Source: CAD feature listing. Evaluate the final solid. Frame: model axes, mm. Face numbers are marked on the shaded views. A direction names the side the tool comes from. Round coordinates to 2 decimals unless told otherwise and drop trailing zeros. Order: outer loops, then holes, each group sorted by start corner. A loop starts at its lowest first (then second) coordinate and runs counter-clockwise, first axis right, second up. Notation, with made-up numbers: (89.5, 15) -> (127.5, 15) arc R16 ccw to (127.5, 24) -> close; hole circle Ø5 at (23, 9). An arc over 180 degrees is marked (long way). Write item = value, one per line. Start each with the question number.
(1) Reachability of the marked faces 1, 2, 3 and 4 from +Z, -Z, +X, -X, +Y, -Y: full face, straight path, thin tool, end or side. Return the list, or none.
(2) Cut plane B-B on x = -3.5. Return the cut outline in (y, z) (3 decimals).
(3) Contact query for flat-ended pins moving along their axis: pin 1 Ø3 at (x, y) = (-2.5, 3) entering from +Z; pin 2 Ø0.7 at (y, z) = (3, 0.5) entering from +X (3 decimals); pin 3 Ø1 at (x, z) = (3.5, 1) entering from -Y (3 decimals); pin 4 Ø0.7 at (y, z) = (-3, 0.5) entering from -X (3 decimals). Output: stop coordinate, or through.
(4) Ray query, line 1 (Y direction, x = -3.5, z = 1.05) (3 decimals); line 2 (X direction, y = -4.75, z = 1.7). Return the intervals inside material, ascending.
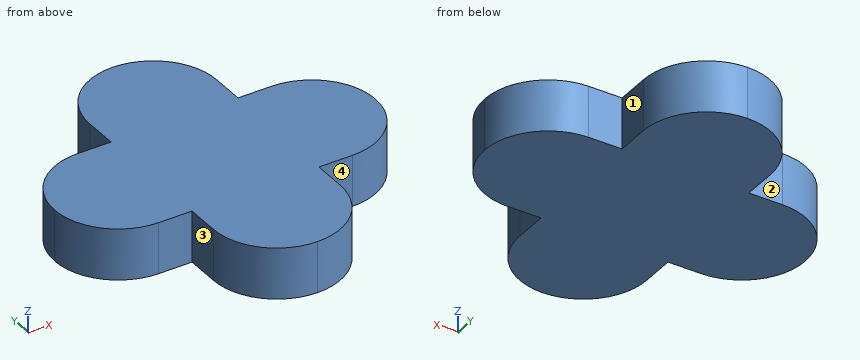
from build123d import *

# Parameters (mm, degrees)
BOSS_EXTRUDE1_DEPTH = 2
FILLET1_R           = 2.475


with BuildPart() as part:
    # Sketch1 → Boss-Extrude1 (new body)
    with BuildSketch(Plane.XY):
        Polygon((2.475, 6.25), (-2.475, 6.25), (-2.475, 2.475), (-6.25, 2.475), (-6.25, -2.475), (-2.475, -2.475), (-2.475, -6.25), (2.475, -6.25), (2.475, -2.475), (6.25, -2.475), (6.25, 2.475), (2.475, 2.475), align=None)
    extrude(amount=BOSS_EXTRUDE1_DEPTH)

    # Fillet1
    fillet1_edges = [part.edges().sort_by_distance(p)[0] for p in [
        (2.475, 6.25, 1),
        (6.25, 2.475, 1),
        (6.25, -2.475, 1),
        (2.475, -6.25, 1),
        (-2.475, -6.25, 1),
        (-6.25, -2.475, 1),
        (-6.25, 2.475, 1),
        (-2.475, 6.25, 1),
    ]]
    fillet(fillet1_edges, radius=FILLET1_R - 0.0001)  # a hair under: the kernel refuses the full size


solid = part.part
Evaluation:
q1.face_1 = +Z, -Z, +X, +Y
q1.face_2 = +Z, -Z, -X, +Y
q1.face_3 = +Z, -Z, -X, -Y
q1.face_4 = +Z, -Z, +X, -Y
q2.outline = (-2.475, 0) -> (2.475, 0) -> (2.475, 2) -> (-2.475, 2) -> close
q3.pin_1 = 2
q3.pin_2 = 2.475
q3.pin_3 = -2.475
q3.pin_4 = -2.475
q4.line_1 = -2.475 to 2.475
q4.line_2 = -2.27 to 2.27
